Could you check a few things on this model? Use its own coordinates, in mm. A direction names the side the tool comes from. Coordinates: 2 decimals unless noted, no trailing zeros. Write each loop counter-clockwise with the first axis right and the second up, starting at its lowest first coordinate (ties: lowest second). Pieces come first, ordered by that corner, then holes. Notation, with made-up numbers: M 24,88.25 L 76,88.25 A21 cw 76,108.25 Z; hole C 41,60.25 d8. An arc over 180 degrees is marked long. Write item = value, one per line.
```python
from build123d import *

# Parameters (mm, degrees)
SKETCH010_W     = 135
SKETCH010_H     = 61
PAD007_DEPTH    = 2
SKETCH011_W     = 8
SKETCH011_H     = 8
PAD008_DEPTH    = 3
SKETCH012_R     = 1.5
POCKET003_DEPTH = 5
SKETCH013_R     = 3
POCKET004_DEPTH = 3
FILLET002_R     = 1
FILLET003_R     = 1


with BuildPart() as part:
    # Sketch010 → Pad007 (new body)
    with BuildSketch(Plane.XY):
        Rectangle(SKETCH010_W, SKETCH010_H)
    extrude(amount=PAD007_DEPTH)

    # Sketch011 (on Face5 of Pad007) → Pad008 (join)
    with BuildSketch(Plane(origin=(0, 0, 0), x_dir=(1, 0, 0), z_dir=(0, 0, -1))):
        with Locations((-63.5, 26.5)):
            Rectangle(SKETCH011_W, SKETCH011_H)
        with Locations((-63.5, -26.5)):
            Rectangle(SKETCH011_W, SKETCH011_H)
        with Locations((63.5, -26.5)):
            Rectangle(SKETCH011_W, SKETCH011_H)
        with Locations((63.5, 26.5)):
            Rectangle(SKETCH011_W, SKETCH011_H)
    extrude(amount=PAD008_DEPTH)

    # Sketch012 (on Face15 of Pad008) → Pocket003 (cut)
    with BuildSketch(Plane.XY.offset(2)):
        with Locations((-63.5, 26.5)):
            Circle(SKETCH012_R)
        with Locations((-63.5, -26.5)):
            Circle(SKETCH012_R)
        with Locations((63.5, 26.5)):
            Circle(SKETCH012_R)
        with Locations((63.5, -26.5)):
            Circle(SKETCH012_R)
    extrude(amount=-POCKET003_DEPTH, mode=Mode.SUBTRACT)

    # Sketch013 (on Face16 of Pocket003) → Pocket004 (cut)
    with BuildSketch(Plane.XY.offset(2)):
        with Locations((-63.5, 26.5)):
            Circle(SKETCH013_R)
        with Locations((-63.5, -26.5)):
            Circle(SKETCH013_R)
        with Locations((63.5, -26.5)):
            Circle(SKETCH013_R)
        with Locations((63.5, 26.5)):
            Circle(SKETCH013_R)
    extrude(amount=-POCKET004_DEPTH, mode=Mode.SUBTRACT)

    # Fillet002
    fillet002_edges = [part.edges().sort_by_distance(p)[0] for p in [
        (67.5, -30.5, -0.5),
        (-67.5, -30.5, -0.5),
        (-67.5, 30.5, -0.5),
        (67.5, 30.5, -0.5),
    ]]
    fillet(fillet002_edges, radius=FILLET002_R)

    # Fillet003
    fillet003_edges = [part.edges().sort_by_distance(p)[0] for p in [
        (59.5, -22.5, -1.5),
        (59.5, 22.5, -1.5),
        (-59.5, 22.5, -1.5),
        (-59.5, -22.5, -1.5),
        (67.5, 22.5, -1.5),
        (59.5, 30.5, -1.5),
        (67.5, -22.5, -1.5),
        (59.5, -30.5, -1.5),
        (-59.5, -30.5, -1.5),
        (-67.5, -22.5, -1.5),
        (-67.5, 22.5, -1.5),
        (-59.5, 30.5, -1.5),
    ]]
    fillet(fillet003_edges, radius=FILLET003_R)


with BuildPart() as part_1:
    # Body002 placement: moved
    add(part.part.moved(Location((0, 0, -24))))


solid = part_1.part
```
Item 1: Imagine slicing it at D-D (x = -20). Write out the boundary of the cut face in (y, z).
Numbers:
outline = M -30.5,-24 L 30.5,-24 L 30.5,-22 L -30.5,-22 Z
Item 2: Imagine slicing it at C-C (y = 6.5). Write out the boundary of the cut face in (x, z), and give its area (3 significant figures).
Numbers:
outline = M -67.5,-24 L 67.5,-24 L 67.5,-22 L -67.5,-22 Z
area = 270 mm²
Item 3: I'm going to push flat-ended pins straight in: P1, Ø3, axis at x = 64, y = 27, coming from the +Z side; P2, Ø5, axis at x = -64.5, y = -25.5, coming from the +Z side; P3, Ø1, axis at x = -12.5, y = -14.5, coming from the -Z side. Where does each tip first touch, or does it pass through?
Numbers:
P1 = -25
P2 = -22
P3 = -24
Item 4: Imagine slicing it at A-A (y = -26.5). Write out the boundary of the cut face in (x, z), and give its area (3 significant figures).
Numbers:
outline = M -67.5,-27 L -65,-27 L -65,-25 L -66.5,-25 L -66.5,-22 L -67.5,-22 Z; M -62,-27 L -59.5,-27 L -59.5,-24 L 59.5,-24 L 59.5,-27 L 62,-27 L 62,-25 L 60.5,-25 L 60.5,-22 L -60.5,-22 L -60.5,-25 L -62,-25 Z; M 65,-27 L 67.5,-27 L 67.5,-22 L 66.5,-22 L 66.5,-25 L 65,-25 Z
area = 270 mm²
Item 5: If we mould it in two halves opening along X, with no side actions, what happens to faces 6 (the face through (-67.5, 0, -23)), 7 (the face through (61.7, -26.6, -27)), 8 (the face through (64.93, 26.95, -25.99))? For each: pulls with the +X half, pulls with the -X half, needs draft (parallel to the pull), parting line crosses it, or undercut.
Numbers:
face_6 = pulls with the -X half
face_7 = needs draft
face_8 = undercut
Item 6: For faces 1 (the face through (-59.5, -26, -25)), 2 (the face through (-64, -22.5, -25)), 3 (the face through (-65.9, 24.7, -23.5)), 4 (the face through (61.7, 26.4, -27)), 5 (the face through (-1, 0, -22)), which set-ups out of +Z, -Z, +X, -X, +Y, -Y let a thin tool reach every point of the face, with its end or its side?
Numbers:
face_1 = -Z, +Y, -Y
face_2 = -Z, +X, -X
face_3 = +Z
face_4 = -Z, +X, -X, +Y, -Y
face_5 = +Z, +X, -X, +Y, -Y
Item 7: Imagine slicing it at B-B (x = -63.5). Write out the boundary of the cut face in (y, z).
Numbers:
outline = M -30.5,-27 L -28,-27 L -28,-25 L -29.5,-25 L -29.5,-22 L -30.5,-22 Z; M -25,-27 L -22.5,-27 L -22.5,-24 L 22.5,-24 L 22.5,-27 L 25,-27 L 25,-25 L 23.5,-25 L 23.5,-22 L -23.5,-22 L -23.5,-25 L -25,-25 Z; M 28,-27 L 30.5,-27 L 30.5,-22 L 29.5,-22 L 29.5,-25 L 28,-25 Z
Item 8: If I drill on line 1 along Y through (x, z) = (63.5, -26.35); line 2 along Y through (x, z) = (-63.5, -23.45); line 3 along Z through (x, y) = (20, -14), over which ranges is the centre line in solid material (lowest first)?
Numbers:
line_1 = -30.5 to -28, -25 to -22.5, 22.5 to 25, 28 to 30.5
line_2 = -30.5 to -29.5, -23.5 to 23.5, 29.5 to 30.5
line_3 = -24 to -22
